```python
from build123d import *

# Parameters (mm, degrees)
SKETCH1_W          = 20
SKETCH1_H          = 4
CHAMFER1_SIZE      = 0.9375
CUT_EXTRUDE4_DEPTH = 3.08
CIRPATTERN1_COUNT  = 6


with BuildPart() as part:
    # Sketch1 → Revolve1 (revolve)
    with BuildSketch(Plane(origin=(0, 0, 0), x_dir=(0, 0, -1), z_dir=(1, 0, 0))):
        with Locations((14.4, 2)):
            Rectangle(SKETCH1_W, SKETCH1_H)
    revolve(axis=Axis((0, 0, -24.4), (0, 0, 1)))

    # Chamfer1
    chamfer1_edges = [part.edges().sort_by_distance(p)[0] for p in [
        (0, -4, -24.4),
    ]]
    chamfer(chamfer1_edges, length=CHAMFER1_SIZE)

    # Sketch7 → Revolve2 (revolve)
    with BuildSketch(Plane(origin=(0, 0, 0), x_dir=(0, 0, -1), z_dir=(1, 0, 0)), mode=Mode.PRIVATE) as revolve2_sk:
        with BuildLine():
            Line((3.74, 7), (4.4, 7))
            Line((4.4, 7), (4.4, 0))
            Line((4.4, 0), (0, 0))
            Line((0, 0), (0, 4))
            ThreePointArc((0, 4), (1.621972026, 5.809208208), (3.74, 7))
        make_face()
    revolve(revolve2_sk.sketch.rotate(Axis((0, 0, 0), (0, 0, -1)), 180), axis=Axis((0, 0, 0), (0, 0, -1)))

    # Sketch11 → Cut-Extrude4 (cut)
    with BuildSketch(Plane.XY):
        with BuildLine():
            Line((0, 0), (-2.771281292, 1.6))
            ThreePointArc((-2.771281292, 1.6), (-2.824655372, 1.386863789), (-2.75740496, 1.177691088))
            ThreePointArc((-2.75740496, 1.177691088), (-2.4, 0), (-2.75740496, -1.177691088))
            ThreePointArc((-2.75740496, -1.177691088), (-2.824655372, -1.386863789), (-2.771281292, -1.6))
            Line((-2.771281292, -1.6), (0, 0))
        make_face()
    cut_extrude4 = extrude(amount=-CUT_EXTRUDE4_DEPTH, mode=Mode.SUBTRACT)

    # CirPattern1: Cut-Extrude4 ×6 about axis
    cirpattern1_axis = Axis((0, 0, 0), (0, 0, 1))
    for i in range(1, CIRPATTERN1_COUNT):
        add(cut_extrude4.rotate(cirpattern1_axis, i * 360 / CIRPATTERN1_COUNT), mode=Mode.SUBTRACT)

    # Cut-Extrude3 cone 1 section (on through the dimple's axis) → Cut-Extrude3 (revolve, cut)
    with BuildSketch(Plane(origin=(0, 0, 0), x_dir=(0, -1, 0), z_dir=(1, 0, 0))):
        Polygon((0, 0), (3.2, 0), (0, 1.847520861), align=None)
    revolve(axis=Axis((0, 0, 0), (0, 0, -1)), mode=Mode.SUBTRACT)


solid = part.part
```
Can you work these out from the model? Positions are in its coordinate system, mm. A direction names the side the tool comes from. Coordinates: 2 decimals unless noted, no trailing zeros. Order: outer loops, then holes, each group sorted by start corner. A loop starts at its lowest first (then second) coordinate and runs counter-clockwise, first axis right, second up. Notation, with made-up numbers: (-8.75, -18.75) -> (33.25, -18.75) arc R17 cw to (33.25, -11.75) -> close; hole circle Ø5 at (50, 87). An arc over 180 degrees is marked (long way). Write each question's results on one line, items separated by ' | '.
Item 1: I'm going to push flat-ended pins straight in: pin 1 Ø4 at (y, z) = (-5.5, -11) entering from +X; pin 2 Ø4 at (x, y) = (3, -3) entering from -Z; pin 3 Ø5 at (y, z) = (-4.5, -12) entering from -X; pin 4 Ø8 at (x, z) = (0, -19) entering from +Y. Where does each tip first touch, or does it pass through?
Results are:
pin 1: x = 1.94 | pin 2: z = -24.4 | pin 3: x = -3.46 | pin 4: y = 4
Item 2: I want a section at A-A, the plane y = 0. Write out the boundary of the cut face in (x, z), then the cut area to 3 significant figures.
Results are:
outline: (-7, -4.4) -> (-4, -4.4) -> (-4, -23.46) -> (-3.06, -24.4) -> (3.06, -24.4) -> (4, -23.46) -> (4, -4.4) -> (7, -4.4) -> (7, -3.74) arc R7.45 ccw to (4, 0) -> (3.2, 0) -> (2.4, -0.46) -> (2.4, -3.08) -> (-2.4, -3.08) -> (-2.4, -0.46) -> (-3.2, 0) -> (-4, 0) arc R7.45 ccw to (-7, -3.74) -> close | area: 197 mm²
Item 3: Which directions (+Z, -Z, +X, -X, +Y, -Y) give clear straight access to the entire face, cutting with the end or side of a thin tool? Please do faces 4 (the face through (2.681, -6.466, -4.075)), 5 (the face through (1.379, 2.43, -0.234)), 6 (the face through (3, -3, -4.4)).
Results are:
face 4: +Z, -Z | face 5: +Z | face 6: -Z
Item 4: If we mould it in two halves opening along X, with no side actions, what happens to faces 1 (the face through (0, 0, -24.4)), 2 (the face through (0, 0, -3.08)), 3 (the face through (3.905, -0.867, -14.065))? For each: +X half, -X half, draft (parallel to the pull), parting line (faces both ways), or undercut.
Results are:
face 1: draft | face 2: undercut | face 3: parting line
Item 5: I want a section at D-D, the plane x = -6. Write out the boundary of the cut face in (y, z).
Results are:
outline: (-3.61, -4.4) -> (3.61, -4.4) -> (3.61, -3.74) arc R4.41 ccw to (-3.61, -3.74) -> close
Item 6: I want a section at B-B, the plane z = -9. Write out the boundary of the cut face in (x, y).
Results are:
outline: circle Ø8 at (0, 0)
Item 7: If I drill on line 1 along Z through (x, y) = (-0.75, -1); line 2 along Y through (x, z) = (3.5, -2.5); line 3 along X through (y, z) = (0, -21.25), over which ranges is the centre line in solid material (lowest first)?
Results are:
line 1: -24.4 to -3.08 | line 2: -5.38 to 5.38 | line 3: -4 to 4
Item 8: I want a section at C-C, the plane x = 5.5. Write out the boundary of the cut face in (y, z).
Results are:
outline: (-4.33, -4.4) -> (4.33, -4.4) -> (4.33, -3.74) arc R5.02 ccw to (-4.33, -3.74) -> close
